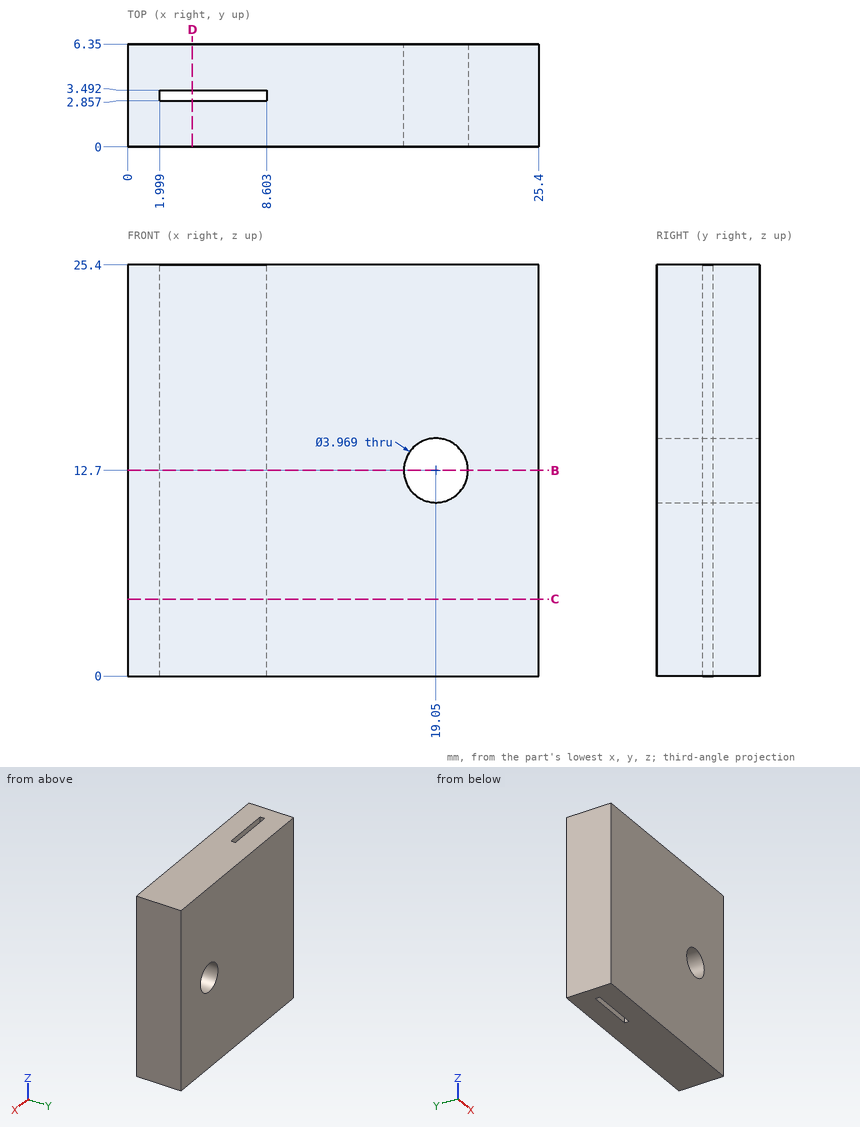
Input: dimensioned drawing with shaded views. Units: mm. Origin: part minimum x, y, z. Round coordinates to 2 decimals unless told otherwise and drop trailing zeros. Loops run counter-clockwise (first coordinate to the right, second up) from the corner with the lowest first, then second, coordinate; pieces in that order, holes last. Notation, with made-up numbers: (55, 88) -> (63, 88) arc R20 cw to (63, 120) -> close; hole circle Ø3 at (9.5, 33). An arc over 180 degrees is marked (long way). Use one line per item in the form item = value. Start each with the question number.
1) Section B-B on z = 12.7. Give the number of separate pieces and of enclosed holes in the cut face, then the cut area to 3 significant figures.
2) First-contact query: P1, Ø2, axis at x = 13, y = 1.5, coming from the -Z side. Flat tip, straight axial feed; report the tip coordinate or a pass-through.
3) Section D-D on x = 4. Output: boundary loops of the cut face in (y, z).
4) Line query: L1, parallel to Z at x = 19.05, y = 3.75 (1 decimal); L2, parallel to Y at x = 5.5, z = 20.75; L3, parallel to X at y = 4.25, z = 11.25 (1 decimal). Output: solid intervals per line, ascending.
5) Section C-C on z = 4.75. Output: boundary loops of the cut face in (x, y).
Response:
q1.separate_pieces = 2
q1.enclosed_holes = 1
q1.area = 132 mm^2
q2.P1 = 0
q3.outline = (0, 0) -> (2.86, 0) -> (2.86, 25.4) -> (0, 25.4) -> close; (3.49, 0) -> (6.35, 0) -> (6.35, 25.4) -> (3.49, 25.4) -> close
q4.L1 = 0 to 10.7, 14.7 to 25.4
q4.L2 = 0 to 2.86, 3.49 to 6.35
q4.L3 = 0 to 17.7, 20.4 to 25.4
q5.outline = (0, 0) -> (25.4, 0) -> (25.4, 6.35) -> (0, 6.35) -> close; hole (2, 2.86) -> (8.6, 2.86) -> (8.6, 3.49) -> (2, 3.49) -> close
